Read the model definition and answer for the solid it produces. Units are mm, in the model's axes. A direction names the side the tool comes from. Coordinates: 2 decimals unless noted, no trailing zeros. Loops run counter-clockwise (first coordinate to the right, second up) from the corner with the lowest first, then second, coordinate; pieces in that order, holes last. Notation, with made-up numbers: M -9.5,-18.5 L 14.5,-18.5 A30 ccw 14.5,6.5 Z; hole C 53.5,-5 d9. An arc over 180 degrees is marked long. Put each result on its own line as item: value.
from build123d import *

# Parameters (mm, degrees)
SKETCH2_W          = 2
SKETCH2_H          = 8
CUT_EXTRUDE1_DEPTH = 3
FILLET1_R          = 0.5
SKETCH3_W          = 3
SKETCH3_H          = 1
CUT_EXTRUDE2_DEPTH = 4


with BuildPart() as part:
    # Sketch1 → Revolve1 (revolve)
    with BuildSketch(Plane.XY):
        with BuildLine():
            Line((0, 0), (0, 4))
            Line((0, 4), (9, 4))
            ThreePointArc((9, 4), (9.585786438, 2.585786438), (11, 2))
            Line((11, 2), (34, 2))
            Line((34, 2), (34, 0))
            Line((34, 0), (0, 0))
        make_face()
    revolve(axis=Axis((0, 0, 0), (1, 0, 0)))

    # Sketch2 → Cut-Extrude1 (cut)
    with BuildSketch(Plane.ZY):
        Rectangle(SKETCH2_W, SKETCH2_H)
    extrude(amount=-CUT_EXTRUDE1_DEPTH, mode=Mode.SUBTRACT)

    # Fillet1
    fillet1_edges = [part.edges().sort_by_distance(p)[0] for p in [
        (0, 0, -4),
        (0, 0, 4),
        (9, -4, 0),
    ]]
    fillet(fillet1_edges, radius=FILLET1_R)

    # Sketch3 → Cut-Extrude2 (cut, symmetric)
    with BuildSketch(Plane.XY):
        with Locations((32.5, 1.5)):
            Rectangle(SKETCH3_W, SKETCH3_H)
    extrude(amount=CUT_EXTRUDE2_DEPTH, both=True, mode=Mode.SUBTRACT)


solid = part.part
1) Which of the six approach directions +Z, -Z, +X, -X, +Y, -Y give full straight-line access (tool end or side, diameter ignored) to faces 1 (the flat face through (34, 0, 0)), 2 (the cylindrical face through (22.7, -1.6, -1.2)), 3 (the flat face through (1, 0, -1)), 4 (the flat face through (32, 1, 0)), 5 (the flat face through (0, 0, -2))?
Answer list:
face 1: +Z, -Z, +X, +Y, -Y
face 2: +X
face 3: -X, +Y, -Y
face 4: +Z, -Z, +X, +Y
face 5: +Z, -Z, -X, +Y, -Y
2) Determine the mould class of faces 6 (the flat face through (1, 0, 1)), 7 (the flat face through (31, 1.4, 0)), 8 (the cylindrical face through (4.582, 3.695, -1.532)) for opening direction Z: released by +Z, released by -Z, zero draft, split by the parting line, or undercut.
Answer list:
face 6: undercut
face 7: zero draft
face 8: split by the parting line
3) Given pin 1 Ø0.9 at (x, y) = (1, -1) entering from -Z; pin 2 Ø2.5 at (x, z) = (32, 1) entering from +Y; pin 3 Ø1 at (y, z) = (1.5, 0) entering from -X, each flat-ended and moving along its own axis, determine where each tip first touches the part or whether it passes through.
Answer list:
pin 1: stops at z = -3.96
pin 2: stops at y = 1.98
pin 3: stops at x = 3
4) Find section A-A, the plane x = 20. Write down the section's boundary in (y, z).
Answer list:
outline: C 0,0 d4
5) Straight lines are drawn through the part: line 1 (X direction, y = 3.25, z = -1.5); line 2 (Z direction, x = 2.5, y = -0.75); line 3 (X direction, y = 1.75, z = 0.5). For each, find the intervals that lie inside material, in ascending order. Write a range as [from, to].
Answer list:
line 1: x = [0.01, 9.04]
line 2: z = [-3.93, -1], [1, 3.93]
line 3: x = [3, 31]
